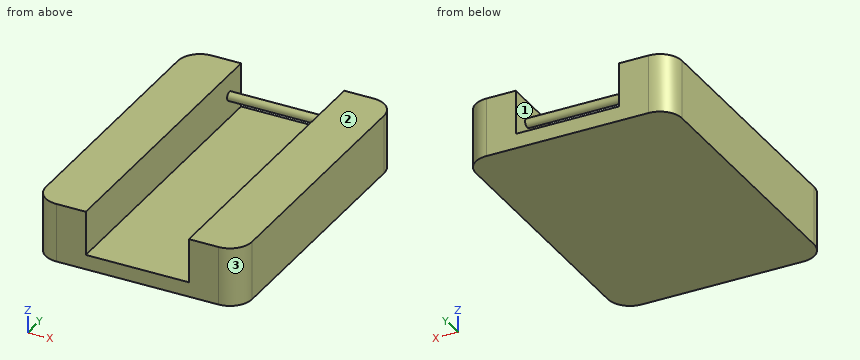
```python
from build123d import *

# Parameters (mm, degrees)
EXTRUDE_1_DEPTH     = 40
CUT_EXTRUDE_1_DEPTH = 30
SKETCH_4_R          = 3
EXTRUDE_2_DEPTH     = 83.650089496


with BuildPart() as part:
    # 草图2 → 凸台-拉伸1 (new body)
    with BuildSketch(Plane.XY):
        with BuildLine():
            Line((0, 100), (-55, 100))
            ThreePointArc((-55, 100), (-65.606601718, 95.606601718), (-70, 85))
            Line((-70, 85), (-70, -85))
            ThreePointArc((-70, -85), (-65.606601718, -95.606601718), (-55, -100))
            Line((-55, -100), (55, -100))
            ThreePointArc((55, -100), (65.606601718, -95.606601718), (70, -85))
            Line((70, -85), (70, 85))
            ThreePointArc((70, 85), (65.606601718, 95.606601718), (55, 100))
            Line((55, 100), (0, 100))
        make_face()
    extrude(amount=EXTRUDE_1_DEPTH)

    # 草图3 → 切除-拉伸1 (cut)
    with BuildSketch(Plane.XY.offset(40)):
        Polygon((0, 100), (-35, 100), (-35, -100), (35, -100), (35, 100), align=None)
    extrude(amount=-CUT_EXTRUDE_1_DEPTH, mode=Mode.SUBTRACT)

    # 草图4 → 凸台-拉伸2 (add)
    with BuildSketch(Plane(origin=(-35, 0, 0), x_dir=(0, 0, -1), z_dir=(1, 0, 0))):
        with Locations(Location((-25, 85, 0), (0, 0, 180))):
            Circle(SKETCH_4_R)
    extrude(amount=EXTRUDE_2_DEPTH)


solid = part.part
```
Here's how the part is built. I have some questions about the finished solid (model axes, mm). Face numbers are marked on the shaded views. Coordinates: 2 decimals unless noted, no trailing zeros. Order: outer loops, then holes, each group sorted by start corner. A loop starts at its lowest first (then second) coordinate and runs counter-clockwise, first axis right, second up. Notation, with made-up numbers: (88.25, 74) - (121.25, 74) arc R14 ccw to (121.25, 81) - close; hole circle Ø1 at (67, 80). An arc over 180 degrees is marked (long way). One line per question, with ' | ' between items. Start each with the question number.
1. I'm going to push flat-ended pins straight in: pin 1 Ø1 at (x, y) = (-18.5, -21.5) entering from +Z; pin 2 Ø4 at (x, z) = (13, 21) entering from +Y. Where does each tip first touch, or does it pass through?
2. If we section it at C-C (y = -32): Write out the boundary of the cut face in (x, z), and give its area (3 significant figures).
3. If we section it at A-A (x = 4): Write out the boundary of the cut face in (y, z).
4. Please list where these lines run through material, in increasing order: line 1 along X through (y, z) = (-32.5, 28.5); line 2 along Z through (x, y) = (-22, 19); line 3 along Y through (x, z) = (57, 23.5). Write a range as [from, to].
5. If we section it at B-B (z = 19): Write out the boundary of the cut face in (x, y).
6. If we mould it in two halves opening along X, with no side actions, what happens to the marked faces 1, 2 and 3? For each: released by +X, released by -X, zero draft, split by the parting line, or undercut.
Model answer:
1) pin 1: stops at z = 10 | pin 2: stops at y = 87.24
2) outline: (-70, 0) - (70, 0) - (70, 40) - (35, 40) - (35, 10) - (-35, 10) - (-35, 40) - (-70, 40) - close | area: 3,500 mm²
3) outline: (-100, 0) - (100, 0) - (100, 10) - (-100, 10) - close; circle Ø6 at (85, 25)
4) line 1: x = [-70, -35], [35, 70] | line 2: z = [0, 10] | line 3: y = [-99.87, 99.87]
5) outline: (-70, -85) arc R15 ccw to (-55, -100) - (-35, -100) - (-35, 100) - (-55, 100) arc R15 ccw to (-70, 85) - close; (35, -100) - (55, -100) arc R15 ccw to (70, -85) - (70, 85) arc R15 ccw to (55, 100) - (35, 100) - close
6) face 1: undercut | face 2: zero draft | face 3: released by +X
